Can you work these out from the model? Positions are in its coordinate system, mm. A direction names the side the tool comes from. Coordinates: 2 decimals unless noted, no trailing zeros. Order: outer loops, then holes, each group sorted by start corner. A loop starts at its lowest first (then second) coordinate and runs counter-clockwise, first axis right, second up. Notation, with made-up numbers: (22, 89.5) -> (65, 89.5) arc R37 ccw to (65, 127.5) -> close; hole circle Ø6 at (78.5, 47). An arc over 180 degrees is marked (long way). Return JSON: item names as keys, results as strings. Group by question number.
1) If we section it at D-D, the plane z = -53: Please give me the cut outline in (x, y).
2) If we section it at A-A, the plane y = 0: Please give me the cut outline in (x, z).
3) For faces 1 (the flat face through (0, 0, 0)), 2 (the flat face through (1.588, 13, -25)), 3 (the flat face through (-1.588, 13, -25)), 4 (the flat face through (-14, -1.588, -57)), which set-ups out of +Z, -Z, +X, -X, +Y, -Y let a thin tool reach every point of the face, with its end or its side?
4) If we section it at B-B, the plane x = 0: Please give me the cut outline in (y, z).
5) If I drill on probe 1 along X at (y, z) = (1.5, -70); probe 2 along X at (y, z) = (0, -64.5); probe 3 along Y at (x, z) = (-0.25, -19.5), over which ranges is the centre line in solid material (lowest first)? Write a range as from..to.
6) If we section it at C-C, the plane z = -28.5: Please give me the cut outline in (x, y), then the cut area to 3 significant figures.
7) For pin 1 (12 mm diameter, centred on y = -8.5, z = -37.5, fed in from -X); pin 2 (0.5 mm diameter, centred on x = 0, y = 13.5, fed in from -Z); pin 3 (4 mm diameter, centred on y = -2.5, z = -30.5, fed in from -X), each with a flat end and sliding along its axis, tell me the tip position at first contact or that it passes through.
Autodesk Inventor part; units mm, degrees
ref_plane "YZ Plane" through (0, 0, 0) normal (1, 0, 0) x (0, 1, 0)
ref_plane "XZ Plane" through (0, 0, 0) normal (0, 1, 0) x (-1, 0, 0)
ref_plane "XY Plane" through (0, 0, 0) normal (0, 0, 1) x (1, 0, 0)
sketch "Sketch1" plane through (0, 0, 0) normal (0, 0, 1) x (1, 0, 0)
  circle A0 centre (0, 0) radius 12.7
  dimension "d0" = 25.4
extrude "Extrusion1" add sketch "Sketch1" against normal blind 76.2
ref_plane "WorkPlaneForFirstKeys" through (0, 0, -19.05) normal (0, 0, 1) x (1, 0, 0)
sketch "Sketch3" plane through (0, 0, -19.05) normal (0, 0, 1) x (1, 0, 0)
  circle A0 centre (0, 0) radius 12.7
  arc A1 (1.5875, 14.199) -> (-1.5875, 14.199) centre (0, 0) ccw
  arc A2 (1.5875, 12.6004) -> (-1.5875, 12.6004) centre (0, 0) ccw
  line L0 (-1.5875, 12.6004) -> (-1.5875, 14.199)
  line L1 (1.5875, 12.6004) -> (1.5875, 14.199)
  line L2 (0, 0) -> (0, 14.2875) construction
  point P0 (-1.5875, 12.6004)
  point P1 (1.5875, 12.6004)
  dimension "d4" = 28.575
  dimension "d6" = 1.5875
  dimension "d7" = 1.5875
extrude "Extrusion2" add sketch "Sketch3" against normal blind 12.7 contours A0 L0 A1 L1
ref_plane "WorkPlaneForSecondKeys" through (0, 0, -50.8) normal (0, 0, 1) x (1, 0, 0)
sketch "Sketch4" plane through (0, 0, -50.8) normal (0, 0, 1) x (1, 0, 0)
  arc A0 (-15.7954, 1.5875) -> (-15.7954, -1.5875) centre (0, 0) ccw
  arc A1 (-12.6004, 1.5875) -> (-12.6004, -1.5875) centre (0, 0) ccw
  line L0 (0, 0) -> (-15.875, 0) construction
  circle A2 centre (0, 0) radius 12.7
  line L1 (-12.6004, -1.5875) -> (-15.7954, -1.5875)
  line L2 (-12.6004, 1.5875) -> (-15.7954, 1.5875)
  dimension "d11" = 31.75
  dimension "d12" = 1.5875
  dimension "d13" = 1.5875
extrude "Extrusion3" add sketch "Sketch4" against normal blind 12.7 contours L2 A1 L1 A0
properties part number "clutch03Shaft"
Result sheet:
{
 "1": {"outline": "(-15.8, -1.59) -> (-12.6, -1.59) arc R12.7 ccw (long way) to (-12.6, 1.59) -> (-15.8, 1.59) arc R15.87 ccw to start"},
 "2": {"outline": "(-15.87, -63.5) -> (-12.7, -63.5) -> (-12.7, -76.2) -> (12.7, -76.2) -> (12.7, 0) -> (-12.7, 0) -> (-12.7, -50.8) -> (-15.87, -50.8) -> close"},
 "3": {"face 1": "+Z, +X, -X, +Y, -Y", "face 2": "+Z, -Z, +X, +Y", "face 3": "+Z, -Z, -X, +Y", "face 4": "+Z, -Z, -X, -Y"},
 "4": {"outline": "(-12.7, -76.2) -> (12.7, -76.2) -> (12.7, -31.75) -> (14.29, -31.75) -> (14.29, -19.05) -> (12.7, -19.05) -> (12.7, 0) -> (-12.7, 0) -> close"},
 "5": {"probe 1": "x = -12.61..12.61", "probe 2": "x = -12.7..12.7", "probe 3": "y = -12.7..14.29"},
 "6": {"outline": "(-1.59, 12.6) arc R12.7 ccw (long way) to (1.59, 12.6) -> (1.59, 14.2) arc R14.29 ccw to (-1.59, 14.2) -> close", "area": "512 mm2"},
 "7": {"pin 1": "stops at x = -12.45", "pin 2": "stops at z = -31.75", "pin 3": "stops at x = -12.69"}
}
